from build123d import *

# Parameters (mm, degrees)
BOSS_EXTRUDE1_DEPTH      = 736.6
BOSS_EXTRUDE1_DEPTH_BACK = 736.6
SKETCH1_W                = 40
SKETCH1_H                = 20
CUT_EXTRUDE1_DEPTH       = 737.939319076
CUT_EXTRUDE1_DEPTH_BACK  = 737.939319076
SKETCH2_W                = 5
SKETCH2_H                = 12
SKETCH2_W_2              = 12
SKETCH2_H_2              = 5


with BuildPart() as part:
    # Sketch1 → Boss-Extrude1 (new, two sides: drawn at the far end of the back side and taken through both)
    with BuildSketch(Plane(origin=(0, 0, 0), x_dir=(1, 0, 0), z_dir=(0, 1, 0)).offset(-BOSS_EXTRUDE1_DEPTH_BACK)):
        Rectangle(SKETCH1_W, SKETCH1_H)
    extrude(amount=BOSS_EXTRUDE1_DEPTH + BOSS_EXTRUDE1_DEPTH_BACK)

    # Sketch2 → Cut-Extrude1 (cut, two sides: drawn at the far end of the back side and taken through both)
    with BuildSketch(Plane(origin=(0, 0, 0), x_dir=(1, 0, 0), z_dir=(0, 1, 0)).offset(-CUT_EXTRUDE1_DEPTH_BACK)):
        with Locations((-10, 10)):
            Rectangle(SKETCH2_W, SKETCH2_H)
        with Locations((-10, -10)):
            Rectangle(SKETCH2_W, SKETCH2_H)
        with Locations((-20, 0)):
            Rectangle(SKETCH2_W_2, SKETCH2_H_2)
        with Locations((10, 10)):
            Rectangle(SKETCH2_W, SKETCH2_H)
        with Locations((20, 0)):
            Rectangle(SKETCH2_W_2, SKETCH2_H_2)
        with Locations((10, -10)):
            Rectangle(SKETCH2_W, SKETCH2_H)
    extrude(amount=CUT_EXTRUDE1_DEPTH + CUT_EXTRUDE1_DEPTH_BACK, mode=Mode.SUBTRACT)


solid = part.part
Input: part model. Units: mm. Frame: model coordinates. Coordinates: 2 decimals unless noted, no trailing zeros. Order: outer loops, then holes, each group sorted by start corner. A loop starts at its lowest first (then second) coordinate and runs counter-clockwise, first axis right, second up.
1. Ray query, line 1 along X through (y, z) = (613, 4.5); line 2 along Z through (x, y) = (17, 233.5); line 3 along Z through (x, y) = (9.5, 269.5). Return the intervals inside material, ascending.
Checked values:
line 1: x = -20 to -12.5, -7.5 to 7.5, 12.5 to 20
line 2: z = -10 to -2.5, 2.5 to 10
line 3: z = -4 to 4
2. Contact query for flat-ended pins moving along their axis: P1, Ø2.5, axis at y = -47, z = -0.5, coming from the -X side; P2, Ø1.5, axis at y = 336, z = -2, coming from the -X side. Output: stop coordinate, or through.
Checked values:
P1: stops at x = -14
P2: stops at x = -20
3. Cut plane A-A, the plane y = 514. Return loops of the section in (x, z).
Checked values:
outline: (-20, -10) - (-12.5, -10) - (-12.5, -4) - (-7.5, -4) - (-7.5, -10) - (7.5, -10) - (7.5, -4) - (12.5, -4) - (12.5, -10) - (20, -10) - (20, -2.5) - (14, -2.5) - (14, 2.5) - (20, 2.5) - (20, 10) - (12.5, 10) - (12.5, 4) - (7.5, 4) - (7.5, 10) - (-7.5, 10) - (-7.5, 4) - (-12.5, 4) - (-12.5, 10) - (-20, 10) - (-20, 2.5) - (-14, 2.5) - (-14, -2.5) - (-20, -2.5) - close
